from build123d import *

# Parameters (mm, degrees)
SKETCH_R        = 25
PAD_DEPTH       = 3
SKETCH001_W     = 5
SKETCH001_H     = 10
PAD001_DEPTH    = 20
SKETCH002_R     = 1.6
POCKET_DEPTH    = 5
SKETCH003_R     = 1.6
SKETCH003_W     = 4
SKETCH003_H     = 13
POCKET001_DEPTH = 35.001
FILLET_R        = 4
FILLET001_R     = 1
FILLET002_R     = 2
POCKET002_DEPTH = 5
POCKET003_DEPTH = 5


with BuildPart() as part:
    # Sketch → Pad (new body)
    with BuildSketch(Plane.XY):
        Circle(SKETCH_R)
    extrude(amount=PAD_DEPTH)

    # Sketch001 (on Face3 of Pad) → Pad001 (join)
    with BuildSketch(Plane.XY.offset(3)):
        with Locations((-7.5, 0)):
            Rectangle(SKETCH001_W, SKETCH001_H)
        with Locations((7.5, 0)):
            Rectangle(SKETCH001_W, SKETCH001_H)
    extrude(amount=PAD001_DEPTH)

    # Sketch002 (on Face3 of Pad001) → Pocket (cut)
    with BuildSketch(Plane.XY.offset(3)):
        Circle(SKETCH002_R)
        with Locations((0, 15)):
            Circle(SKETCH002_R)
    extrude(amount=-POCKET_DEPTH, mode=Mode.SUBTRACT)

    # Sketch003 (on Face8 of Pocket) → Pocket001 (cut, through all)
    with BuildSketch(Plane(origin=(-10, 0, 0), x_dir=(0, -1, 0), z_dir=(-1, 0, 0))):
        with Locations((0, 20)):
            Circle(SKETCH003_R)
        with Locations((0, 9.5)):
            Rectangle(SKETCH003_W, SKETCH003_H)
    extrude(amount=-POCKET001_DEPTH, mode=Mode.SUBTRACT)

    # Fillet
    fillet_edges = [part.edges().sort_by_distance(p)[0] for p in [
        (-7.5, 5, 23),
        (-7.5, -5, 23),
        (7.5, -5, 23),
        (7.5, 5, 23),
    ]]
    fillet(fillet_edges, radius=FILLET_R)

    # Fillet001
    fillet001_edges = [part.edges().sort_by_distance(p)[0] for p in [
        (7.5, -2, 16),
        (-7.5, -2, 16),
        (-7.5, 2, 16),
        (7.5, 2, 16),
    ]]
    fillet(fillet001_edges, radius=FILLET001_R)

    # Fillet002
    fillet002_edges = [part.edges().sort_by_distance(p)[0] for p in [
        (-25, 0, 3),
    ]]
    fillet(fillet002_edges, radius=FILLET002_R)

    # Sketch004 (on Face1 of Fillet002) → Pocket002 (cut)
    with BuildSketch(Plane.XY.offset(3)):
        with BuildLine():
            ThreePointArc((0, -16.6), (16.6, 0), (0, 16.6))
            Line((0, 16.6), (0, 13.4))
            ThreePointArc((0, -13.4), (13.4, 0), (0, 13.4))
            Line((0, -13.4), (0, -16.6))
        make_face()
    extrude(amount=-POCKET002_DEPTH, mode=Mode.SUBTRACT)

    # Sketch005 (on Face1 of Pocket002) → Pocket003 (cut)
    with BuildSketch(Plane.XY.offset(3)):
        with BuildLine():
            ThreePointArc((0, -13.4), (-1.6, -15), (0, -16.6))
            Line((0, -13.4), (0, -16.6))
        make_face()
    extrude(amount=-POCKET003_DEPTH, mode=Mode.SUBTRACT)


solid = part.part
For this review, take the finished solid that the model builds, in its own axes (mm). A direction names the side the tool comes from. Give positions to 0.01 mm unless a question says otherwise; leave off trailing zeros. Loops run counter-clockwise (first coordinate to the right, second up) from the corner with the lowest first, then second, coordinate; pieces in that order, holes last.
Item 1: Draft analysis for pull direction Y (two halves, no side actions). For faces 6 (the flat face through (-8, 5, 11)), 7 (the cylindrical face through (13.397, -0.295, 1.521)), 8 (the cylindrical face through (-7.465, -3.859, 21.797)), 9 (the flat face through (-8, 0, 23)), state which applies: +Y half, -Y half, draft (parallel to the pull), parting line (faces both ways), or undercut.
Item 2: Insertion check: pin 1 (1.5 mm diameter, centred on x = 7, z = 8.5, fed in from -Y); pin 2 (1.5 mm diameter, centred on x = 7.5, z = 12, fed in from +Y); pin 3 (2.5 mm diameter, centred on x = 0, y = 0, fed in from -Z); pin 4 (2 mm diameter, centred on x = 12.5, y = -2, fed in from +Z). Each pin has a flat end and moves straight along its axis. Give the tip position at first contact, or say it passes through.
Item 3: Tool access review of faces 1 (the flat face through (-8, -5, 11)), 2 (the flat face through (7, 5, 11)), 3 (the flat face through (7, -2, 9)), 4 (the cylindrical face through (-1.6, 15, 1.5)), 5 (the flat face through (5, 2.2, 12.9)): name each direction out of +Z, -Z, +X, -X, +Y, -Y from which nothing blocks a thin tool from reaching the whole face with its end or side.
Item 4: Take a section at C-C, the plane x = -1. Give the number of separate pieces and of enclosed holes in the cut face, and give its area (3 significant figures).
Item 5: Take a section at B-B, the plane z = 13.25. State the section outline as (x, y) points.
Item 6: For line 1 along Z through (x, y) = (7.55, 0); line 2 along X through (y, z) = (-4.5, 15.25); line 3 along Z through (x, y) = (-15, 2), list the stretches that pass through material, from the lowest coordinate up.
Item 7: Take a section at A-A, the plane z = 17.25. State the section outline as (x, y) points, and give its area (3 significant figures).
Calculated:
1. face 6: +Y half
1. face 7: undercut
1. face 8: -Y half
1. face 9: draft
2. pin 1: stops at y = -5
2. pin 2: stops at y = 5
2. pin 3: passes through
2. pin 4: stops at z = 3
3. face 1: +Z, +X, -X, -Y
3. face 2: +Z, +X, -X, +Y
3. face 3: +X, -X
3. face 4: +Z, -Z
3. face 5: +Z, +Y, -Y
4. separate pieces: 4
4. enclosed holes: 0
4. area: 126 mm2
5. outline: (-10, -5) - (-5, -5) - (-5, -2) - (-10, -2) - close; (-10, 2) - (-5, 2) - (-5, 5) - (-10, 5) - close; (5, -5) - (10, -5) - (10, -2) - (5, -2) - close; (5, 2) - (10, 2) - (10, 5) - (5, 5) - close
6. line 1: z = 0 to 3, 16 to 18.4, 21.6 to 23
6. line 2: x = -10 to -5, 5 to 10
6. line 3: z = 0 to 3
7. outline: (-10, -5) - (-5, -5) - (-5, 5) - (-10, 5) - close; (5, -5) - (10, -5) - (10, 5) - (5, 5) - close
7. area: 100 mm2
